from build123d import *

# Parameters (mm, degrees)
BOSS_EXTRUDE1_DEPTH = 60
CUT_EXTRUDE9_DEPTH  = 25
SKETCH5_OUTSIDE_W   = 324.786
SKETCH5_OUTSIDE_H   = 308.698
SKETCH5_OUTSIDE_R   = 52.224812322
CUT_EXTRUDE10_DEPTH = 100.545634426
CUT_EXTRUDE10_DRAFT = -40
SKETCH6_R           = 25
CUT_EXTRUDE11_DEPTH = 100.545634426


with BuildPart() as part:
    # Sketch1 → Boss-Extrude1 (new body)
    with BuildSketch(Plane(origin=(0, 0, 0), x_dir=(1, 0, 0), z_dir=(0, 1, 0))):
        Polygon((30.022213998, -52), (60.044427996, 0), (30.022213998, 52), (-30.022213998, 52), (-60.044427996, 0), (-30.022213998, -52), align=None)
    extrude(amount=BOSS_EXTRUDE1_DEPTH)

    # Sketch2 → Cut-Extrude9 (cut)
    with BuildSketch(Plane(origin=(0, 60, 0), x_dir=(1, 0, 0), z_dir=(0, 1, 0))):
        with BuildLine():
            Line((5, 52), (-5, 52))
            Line((-5, 52), (-5, 24.494897428))
            ThreePointArc((-5, 24.494897428), (0, 25), (5, 24.494897428))
            Line((5, 24.494897428), (5, 52))
        make_face()
        with BuildLine():
            ThreePointArc((5, -24.494897428), (0, -25), (-5, -24.494897428))
            Line((-5, -24.494897428), (-5, -52))
            Line((-5, -52), (5, -52))
            Line((5, -52), (5, -24.494897428))
        make_face()
        with BuildLine():
            Line((42.533320997, 30.330127019), (18.713203436, 16.577575733))
            ThreePointArc((18.713203436, 16.577575733), (21.650635095, 12.5), (23.713203436, 7.917321695))
            Line((23.713203436, 7.917321695), (47.533320997, 21.669872981))
            Line((47.533320997, 21.669872981), (42.533320997, 30.330127019))
        make_face()
        with BuildLine():
            ThreePointArc((-23.713203436, 7.917321695), (-21.650635095, 12.5), (-18.713203436, 16.577575733))
            Line((-18.713203436, 16.577575733), (-42.533320997, 30.330127019))
            Line((-42.533320997, 30.330127019), (-47.533320997, 21.669872981))
            Line((-47.533320997, 21.669872981), (-23.713203436, 7.917321695))
        make_face()
        with BuildLine():
            ThreePointArc((-18.713203436, -16.577575733), (-21.650635095, -12.5), (-23.713203436, -7.917321695))
            Line((-23.713203436, -7.917321695), (-47.533320997, -21.669872981))
            Line((-47.533320997, -21.669872981), (-42.533320997, -30.330127019))
            Line((-42.533320997, -30.330127019), (-18.713203436, -16.577575733))
        make_face()
        with BuildLine():
            Line((47.533320997, -21.669872981), (23.713203436, -7.917321695))
            ThreePointArc((23.713203436, -7.917321695), (21.650635095, -12.5), (18.713203436, -16.577575733))
            Line((18.713203436, -16.577575733), (42.533320997, -30.330127019))
            Line((42.533320997, -30.330127019), (47.533320997, -21.669872981))
        make_face()
    extrude(amount=-CUT_EXTRUDE9_DEPTH, mode=Mode.SUBTRACT)


with BuildPart() as cut_extrude10_tool:
    # Sketch5 outside → Cut-Extrude10 (with draft: the straight prism first)
    with BuildSketch(Plane(origin=(0, 60, 0), x_dir=(1, 0, 0), z_dir=(0, 1, 0))):
        Rectangle(SKETCH5_OUTSIDE_W, SKETCH5_OUTSIDE_H)
        Circle(SKETCH5_OUTSIDE_R, mode=Mode.SUBTRACT)
    extrude(amount=-CUT_EXTRUDE10_DEPTH)
    # Cut-Extrude10: the draft: its side faces are tilted about the plane it starts from
    cut_extrude10_sides = [cut_extrude10_tool.faces().sort_by_distance(p)[0] for p in [
        (0, 9.727182787, 154.349),
        (162.393, 9.727182787, 0),
        (0, 9.727182787, -154.349),
        (-162.393, 9.727182787, 0),
        (-52.224812322, 9.727182787, 0),
    ]]
    draft(cut_extrude10_sides, Plane(origin=(0, 60, 0), x_dir=(1, 0, 0), z_dir=(0, 1, 0)), CUT_EXTRUDE10_DRAFT)


with BuildPart() as part_1:
    add(part.part)

    # Cut-Extrude10: cut by cut_extrude10_tool
    add(cut_extrude10_tool.part, mode=Mode.SUBTRACT)

    # Sketch6 → Cut-Extrude11 (cut, through all)
    with BuildSketch(Plane(origin=(0, 60, 0), x_dir=(1, 0, 0), z_dir=(0, 1, 0))):
        with Locations(Location((0, 0, 0), (0, 0, 270))):
            Circle(SKETCH6_R)
    extrude(amount=-CUT_EXTRUDE11_DEPTH, mode=Mode.SUBTRACT)


solid = part_1.part
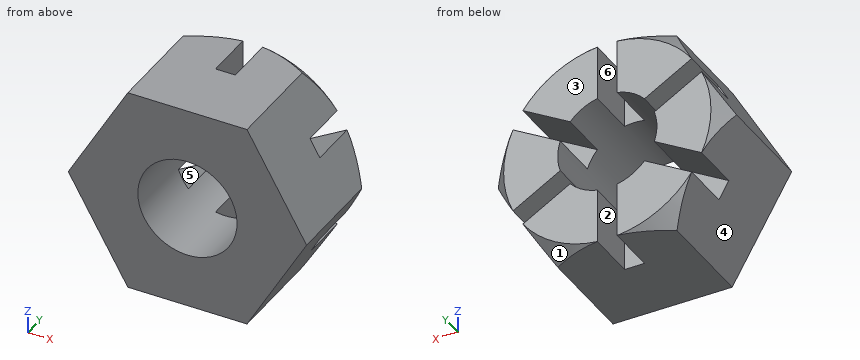
The listing builds one solid part. Answer for the finished solid, in the listing's coordinates (mm). Face numbers are marked on the shaded views. A direction names the side the tool comes from. Give positions to 0.01 mm unless a question says otherwise; leave off trailing zeros. Write each loop counter-clockwise with the first axis right and the second up, starting at its lowest first coordinate (ties: lowest second). Pieces come first, ordered by that corner, then holes. Notation, with made-up numbers: (58, -27) -> (88, -27) arc R21 cw to (88, -6) -> close; hole circle Ø10 at (-20.75, 38.5). An arc over 180 degrees is marked (long way). One line per question, with ' | ' between items. Start each with the question number.
1. Section C-C (z = 27) is taken. Determine the outline of the cut face in (x, y).
2. For a pull along X with two mould halves and no side action, classify the marked faces 1, 2 and 3 as pulls with the +X half, pulls with the -X half, needs draft (parallel to the pull), parting line crosses it, or undercut.
3. Given pin 1 Ø1 at (y, z) = (42.5, -29.5) entering from -X; pin 2 Ø3 at (x, z) = (0.5, -32.5) entering from +Y; pin 3 Ø7.5 at (y, z) = (50, -38.5) entering from +X; pin 4 Ø1 at (x, z) = (8.5, -21) entering from -Y, each flat-ended and moving along its own axis, determine where each tip first touches the part or whether it passes through.
4. For the marked faces 4, 5 and 6, determine the directions among +Z, -Z, +X, -X, +Y, -Y from which every point of the face is accessible in a straight line to the end or side of a thin tool.
5. Section B-B (y = 29.5) is taken. Determine the outline of the cut face in (x, z), plus the area to 3 significant figures.
6. Find the intervals of material crossed by probe 1 along Z at (x, y) = (0, 23); probe 2 along Z at (x, y) = (38, 39); probe 3 along Z at (x, y) = (-12.5, 19.5), in increasing order.
7. Section A-A (x = 0) is taken. Determine the outline of the cut face in (y, z).
Response values:
1) outline: (-44.46, 0) -> (44.46, 0) -> (44.46, 35) -> (36.77, 35) -> (36.77, 60) -> (5, 60) -> (5, 35) -> (-5, 35) -> (-5, 60) -> (-36.77, 60) -> (-36.77, 35) -> (-44.46, 35) -> close
2) face 1: pulls with the +X half | face 2: undercut | face 3: needs draft
3) pin 1: x = -41.96 | pin 2: y = 35 | pin 3: x = 39.98 | pin 4: through
4) face 4: -Z, -X, +Y, -Y | face 5: +Y | face 6: +Z, -Z, +Y
5) outline: (-60.04, 0) -> (-30.02, -52) -> (30.02, -52) -> (60.04, 0) -> (30.02, 52) -> (-30.02, 52) -> close; hole circle Ø50 at (0, 0) | area: 7,400 mm2
6) probe 1: -52 to -25, 25 to 52 | probe 2: -38.18 to -27.71, -16.17 to 16.17, 27.71 to 38.18 | probe 3: -52 to -21.65, 21.65 to 52
7) outline: (0, -52) -> (35, -52) -> (35, -25) -> (0, -25) -> close; (0, 25) -> (35, 25) -> (35, 52) -> (0, 52) -> close
